```python
from build123d import *

# Parameters (mm, degrees)
SKETCH1_W              = 101.6
SKETCH1_H              = 38.1
BOSS_EXTRUDE1_DEPTH    = 12.7
F_4_0MM_DOWEL_HOLE1_D  = 4
SKETCH7_R              = 2.9972
CUT_EXTRUDE1_DEPTH     = 5.08
F_10_32_TAPPED_HOLE1_D = 4.0386


with BuildPart() as part:
    # Sketch1 → Boss-Extrude1 (new body)
    with BuildSketch(Plane.XY):
        Rectangle(SKETCH1_W, SKETCH1_H)
    extrude(amount=BOSS_EXTRUDE1_DEPTH)

    # Ø4.0mm Dowel Hole1 (through all)
    with Locations(Plane.XY.offset(12.7)):
        with Locations((0, 9.99998), (0, -9.99998)):
            Hole(F_4_0MM_DOWEL_HOLE1_D / 2)

    # Sketch7 → Cut-Extrude1 (cut)
    with BuildSketch(Plane.XY.offset(12.7)):
        with Locations((0, -10.079486129)):
            Circle(SKETCH7_R)
        with Locations((0, 9.99998)):
            Circle(SKETCH7_R)
    extrude(amount=-CUT_EXTRUDE1_DEPTH, mode=Mode.SUBTRACT)

    # #10-32 Tapped Hole1 (through all)
    with Locations(Plane(origin=(0, 19.05, 0), x_dir=(1, 0, 0), z_dir=(0, 1, 0))):
        with Locations((38.1, -6.35), (12.7, -6.35), (-12.7, -6.35), (-38.1, -6.35)):
            Hole(F_10_32_TAPPED_HOLE1_D / 2)


solid = part.part
```
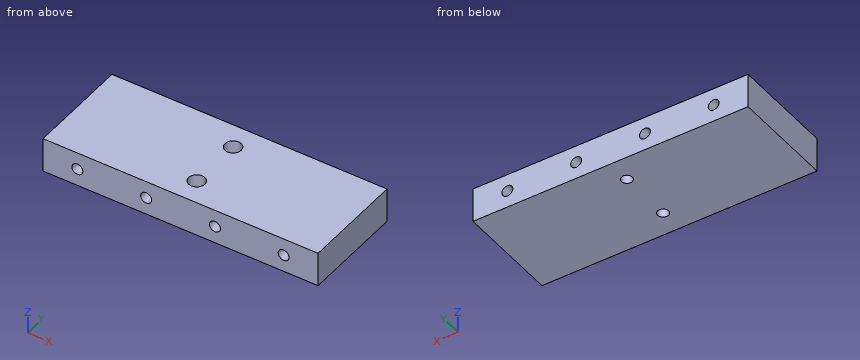
Design review of the part built by this model. Coordinates are the model's own, in mm. Round coordinates to 2 decimals unless told otherwise and drop trailing zeros. Order: outer loops, then holes, each group sorted by start corner. A loop starts at its lowest first (then second) coordinate and runs counter-clockwise, first axis right, second up. Notation, with made-up numbers: (33.5, 50.25) - (38.5, 50.25) arc R10 ccw to (38.5, 69.25) - close; hole circle Ø9 at (46.5, 40). An arc over 180 degrees is marked (long way). Return JSON: item names as keys, results as strings.
Q1. Consider section B-B on y = -1.5. Write out the cut boundary in (x, z), plus the area to 3 significant figures.
Computed values:
{"outline": "(-50.8, 0) - (50.8, 0) - (50.8, 12.7) - (-50.8, 12.7) - close; hole circle Ø4.04 at (-38.1, 6.35); hole circle Ø4.04 at (-12.7, 6.35); hole circle Ø4.04 at (12.7, 6.35); hole circle Ø4.04 at (38.1, 6.35)", "area": "1,240 mm2"}
Q2. Wall thickness on L1, parallel to Y at x = 0, z = 3; L2, parallel to Y at x = 0, z = 11; L3, parallel to X at y = 10, z = 2.5: over which ranges is each line inside the solid? List them lowest first. Write a range as [from, to].
Computed values:
{"L1": "y = [-19.05, -12], [-8, 8], [12, 19.05]", "L2": "y = [-19.05, -13.08], [-7.08, 7], [13, 19.05]", "L3": "x = [-50.8, -2], [2, 50.8]"}
Q3. Consider section A-A on z = 5.25. Write out the cut boundary in (x, y).
Computed values:
{"outline": "(-50.8, -19.05) - (-39.79, -19.05) - (-39.79, 19.05) - (-50.8, 19.05) - close; (-36.41, -19.05) - (-14.39, -19.05) - (-14.39, 19.05) - (-36.41, 19.05) - close; (-11.01, -19.05) - (11.01, -19.05) - (11.01, 19.05) - (-11.01, 19.05) - close; (14.39, -19.05) - (36.41, -19.05) - (36.41, 19.05) - (14.39, 19.05) - close; (39.79, -19.05) - (50.8, -19.05) - (50.8, 19.05) - (39.79, 19.05) - close; hole circle Ø4 at (0, -10); hole circle Ø4 at (0, 10)"}
Q4. For pin 1 Ø2.5 at (x, y) = (0, -10) entering from +Z; pin 2 Ø3 at (x, y) = (0.5, -9) entering from +Z, all flat-tipped, find the tip position at first contact; note any pin that passes through.
Computed values:
{"pin 1": "passes through", "pin 2": "stops at z = 7.62"}
Q5. Consider section C-C on x = 12.7. Write out the cut boundary in (y, z).
Computed values:
{"outline": "(-19.05, 0) - (19.05, 0) - (19.05, 4.33) - (-19.05, 4.33) - close; (-19.05, 8.37) - (19.05, 8.37) - (19.05, 12.7) - (-19.05, 12.7) - close"}
